from build123d import *

# Parameters (mm, degrees)
EXTRUDE_1_DEPTH   = 2
HOLE_WIZARD_M81_D = 9
CHAMFER_1_SIZE    = 2


with BuildPart() as part:
    # Эскиз1 → Бобышка-Вытянуть1 (new body)
    with BuildSketch(Plane(origin=(0, 0, 0), x_dir=(1, 0, 0), z_dir=(0, 0, -1))):
        Polygon((0, 0), (0, 150), (150, 150), (150, 100), (50, 0), align=None)
    extrude(amount=EXTRUDE_1_DEPTH)

    # Отверстие с зазором M81 (through all)
    with Locations(Plane(origin=(0, 0, -2), x_dir=(1, 0, 0), z_dir=(0, 0, -1))):
        with Locations((75, 125), (25, 125), (25, 75), (25, 25), (125, 125), (75, 75)):
            Hole(HOLE_WIZARD_M81_D / 2)

    # Фаска1
    chamfer_1_edges = [part.edges().sort_by_distance(p)[0] for p in [
        (0, 0, -1),
        (0, -150, -1),
        (150, -150, -1),
    ]]
    chamfer(chamfer_1_edges, length=CHAMFER_1_SIZE)


solid = part.part
Here's how the part is built. I have some questions about the finished solid (model axes, mm). Coordinates: 2 decimals unless noted, no trailing zeros. Order: outer loops, then holes, each group sorted by start corner. A loop starts at its lowest first (then second) coordinate and runs counter-clockwise, first axis right, second up. Notation, with made-up numbers: M 67,63.25 L 105,63.25 A18 ccw 105,92.25 Z; hole C 79,11.5 d11. An arc over 180 degrees is marked long. Answer as CSV lines item,"result". Start each with the question number.
1. I need wall thicknesses on line 1 (X direction, y = -125, z = -0.9); line 2 (Y direction, x = 25, z = -1.25); line 3 (Y direction, x = 75, z = -0.75). Which ranges of each line are inside material? Lowest first, please. Write a range as [from, to].
2. I want a section at B-B, the plane y = -25. Write out the boundary of the cut face in (x, z).
3. I want a section at C-C, the plane z = -1.3. Write out the boundary of the cut face in (x, y).
4. For pin 1 (8 mm diameter, centred on x = 25, y = -25, fed in from +Z), with a flat end and sliding along its axis, tell me the tip position at first contact or that it passes through.
5. I want a section at D-D, the plane x = 125. Write out the boundary of the cut face in (y, z), and give its area (3 significant figures).
6. I want a section at A-A, the plane x = 75. Write out the boundary of the cut face in (y, z).
Recorded:
1,line 1,"x = [0, 20.5], [29.5, 70.5], [79.5, 120.5], [129.5, 150]"
1,line 2,"y = [-150, -129.5], [-120.5, -79.5], [-70.5, -29.5], [-20.5, 0]"
1,line 3,"y = [-150, -129.5], [-120.5, -79.5], [-70.5, -25]"
2,outline,"M 0,-2 L 20.5,-2 L 20.5,0 L 0,0 Z; M 29.5,-2 L 75,-2 L 75,0 L 29.5,0 Z"
3,outline,"M 0,-148 L 2,-150 L 148,-150 L 150,-148 L 150,-100 L 50,0 L 2,0 L 0,-2 Z; hole C 25,-125 d9; hole C 25,-75 d9; hole C 25,-25 d9; hole C 75,-125 d9; hole C 75,-75 d9; hole C 125,-125 d9"
4,pin 1,"passes through"
5,outline,"M -150,-2 L -129.5,-2 L -129.5,0 L -150,0 Z; M -120.5,-2 L -75,-2 L -75,0 L -120.5,0 Z"
5,area,"132 mm2"
6,outline,"M -150,-2 L -129.5,-2 L -129.5,0 L -150,0 Z; M -120.5,-2 L -79.5,-2 L -79.5,0 L -120.5,0 Z; M -70.5,-2 L -25,-2 L -25,0 L -70.5,0 Z"
